For this review, use the dimensioned drawing (mm, ordinates from the lowest corner) and the shaded views. Coordinates: 2 decimals unless noted, no trailing zeros. Loops run counter-clockwise (first coordinate to the right, second up) from the corner with the lowest first, then second, coordinate; pieces in that order, holes last.
1. Take a section at D-D, the plane x = 34.5. State the section outline as (y, z) points (1 decimal).
2. Take a section at C-C, the plane y = 2.9. State the section outline as (x, z) points (1 decimal).
3. To check wall thickness, follow probe 1 along Z at (x, y) = (21.5, 3.9) (1 decimal); probe 2 along X at (y, z) = (1.7, 45.5) (1 decimal); probe 3 along Z at (x, y) = (45, 1.3) (1 decimal). State the ranges of each line that lie inside material, in increasing order.
4. Take a section at A-A, the plane x = 21.5. State the section outline as (y, z) points (1 decimal).
5. Clearance check with flat-ended pins moving along their axes: P1, Ø2.5, axis at y = 2.5, z = 35.5, coming from the +X side; P2, Ø1.5, axis at x = 21.5, y = 3.5, coming from the +Z side; P3, Ø2, axis at y = 2.5, z = 16.5, coming from the +X side; P4, Ø1, axis at x = 28, z = 22, coming from the -Y side. State where each tip first meets the part, or that it passes through.
6. Take a section at B-B, the plane z = 40.5. State the section outline as (x, y) points (1 decimal).
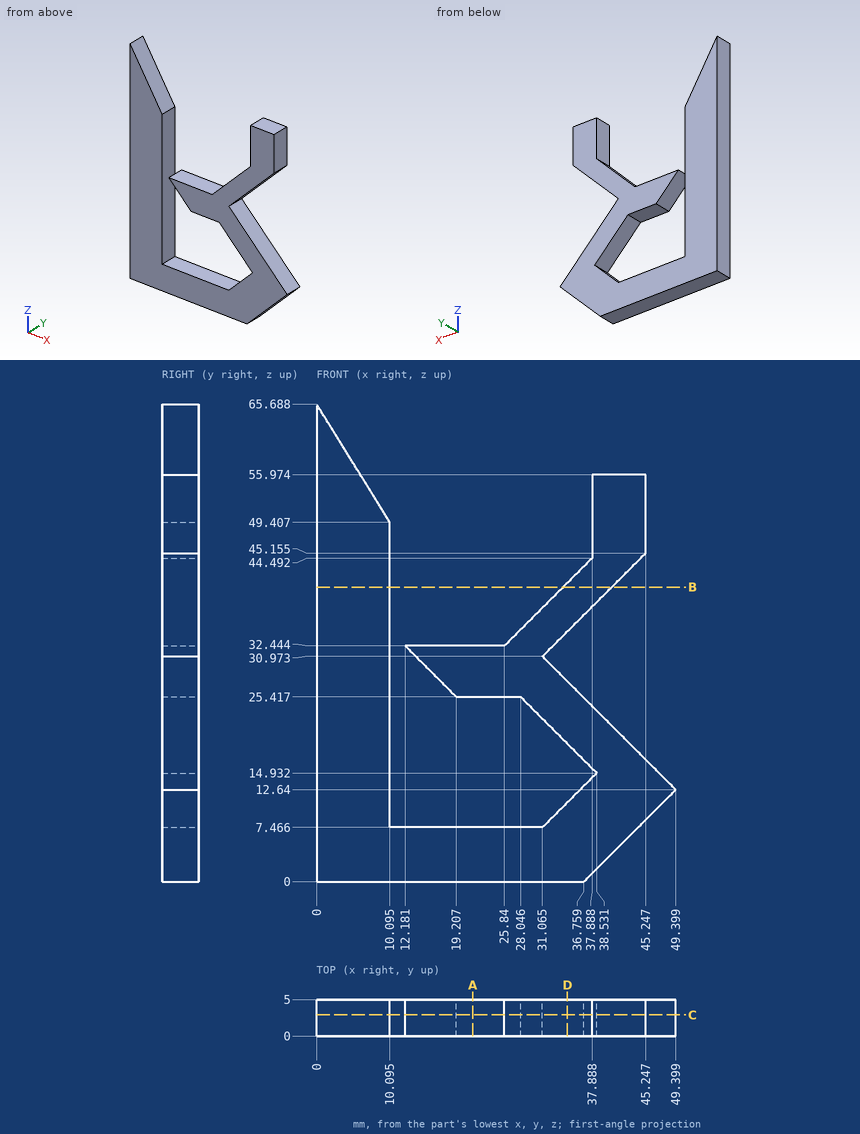
Results list:
1. outline: (0, 0) - (5, 0) - (5, 10.9) - (0, 10.9) - close; (0, 19) - (5, 19) - (5, 27.5) - (0, 27.5) - close; (0, 34.4) - (5, 34.4) - (5, 41.1) - (0, 41.1) - close
2. outline: (0, 0) - (36.8, 0) - (49.4, 12.6) - (31.1, 31) - (45.2, 45.2) - (45.2, 56) - (37.9, 56) - (37.9, 44.5) - (25.8, 32.4) - (12.2, 32.4) - (19.2, 25.4) - (28, 25.4) - (38.5, 14.9) - (31.1, 7.5) - (10.1, 7.5) - (10.1, 49.4) - (0, 65.7) - close
3. probe 1: z = 0 to 7.5, 25.4 to 32.4
3. probe 2: x = 0 to 10.1, 37.9 to 45.2
3. probe 3: z = 8.2 to 17, 44.9 to 56
4. outline: (0, 0) - (5, 0) - (5, 7.5) - (0, 7.5) - close; (0, 25.4) - (5, 25.4) - (5, 32.4) - (0, 32.4) - close
5. P1: stops at x = 36.84
5. P2: stops at z = 32.44
5. P3: stops at x = 46.54
5. P4: passes through
6. outline: (0, 0) - (10.1, 0) - (10.1, 5) - (0, 5) - close; (33.9, 0) - (40.6, 0) - (40.6, 5) - (33.9, 5) - close
